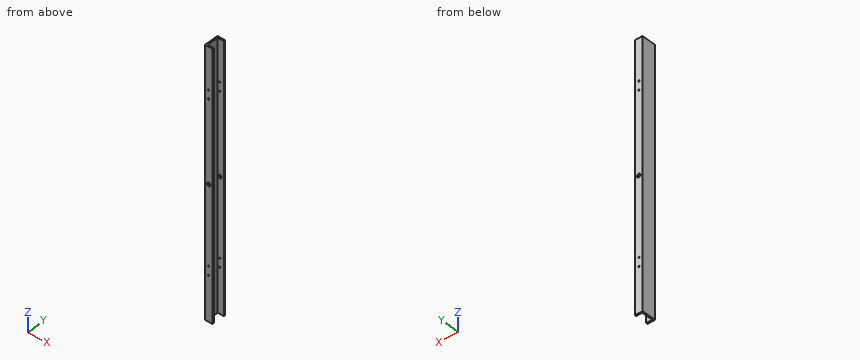
from build123d import *

# Parameters (mm, degrees)
BOSS_EXTRUDE1_DEPTH = 1360
SKETCH2_R           = 3.5
SKETCH2_R_2         = 9
CUT_EXTRUDE1_DEPTH  = 814.403343981


with BuildPart() as part:
    # Sketch1 → Boss-Extrude1 (new body)
    with BuildSketch(Plane.XY.offset(-680)):
        Polygon((-440, 550), (-440, 625), (-400, 625), (-400, 617), (-432, 617), (-432, 558), (-400, 558), (-400, 550), align=None)
    extrude(amount=BOSS_EXTRUDE1_DEPTH)

    # Sketch2 → Cut-Extrude1 (cut, through all)
    with BuildSketch(Plane(origin=(0, 625, 0), x_dir=(1, 0, 0), z_dir=(0, 1, 0))):
        with Locations(Location((-421, -467, 0), (0, 0, 270))):
            Circle(SKETCH2_R)
        with Locations(Location((-421, -422, 0), (0, 0, 270))):
            Circle(SKETCH2_R)
        with Locations(Location((-420, 0, 0), (0, 0, 270))):
            Circle(SKETCH2_R_2)
        with Locations(Location((-421, 450, 0), (0, 0, 270))):
            Circle(SKETCH2_R)
        with Locations(Location((-421, 405, 0), (0, 0, 270))):
            Circle(SKETCH2_R)
    extrude(amount=-CUT_EXTRUDE1_DEPTH, mode=Mode.SUBTRACT)


solid = part.part
The model under review builds one solid part; all positions refer to its coordinate system, in mm. Coordinates: 2 decimals unless noted, no trailing zeros. Loops run counter-clockwise (first coordinate to the right, second up) from the corner with the lowest first, then second, coordinate; pieces in that order, holes last. Notation, with made-up numbers: M -10.5,-29.75 L 32.5,-29.75 A17 ccw 32.5,1.25 Z; hole C -23,75 d4. An arc over 180 degrees is marked long. Put each result on its own line as item: value. Start each with the question number.
Q1. Add section B-B (y = 597.5). Write out the cut boundary in (x, z).
Q2. Clearance check with flat-ended pins moving along their axes: pin 1 (3 mm diameter, centred on y = 602.5, z = -86, fed in from +X); pin 2 (9 mm diameter, centred on x = -421, z = -450, fed in from +Y). State where each tip first meets the part, or that it passes through.
Q3. Add section A-A (z = 230). Write out the cut boundary in (x, y).
Q4. Wall thickness on line 1 (Z direction, x = -421, y = 621.25); line 2 (X direction, y = 619.75, z = -450); line 3 (Y direction, x = -404.5, z = 479.5): over which ranges is each line inside the solid? List them lowest first.
Answers:
1. outline: M -440,-680 L -432,-680 L -432,680 L -440,680 Z
2. pin 1: stops at x = -432
2. pin 2: stops at y = 625
3. outline: M -440,550 L -400,550 L -400,558 L -432,558 L -432,617 L -400,617 L -400,625 L -440,625 Z
4. line 1: z = -680 to -453.5, -446.5 to -408.5, -401.5 to -8.94, 8.94 to 418.5, 425.5 to 463.5, 470.5 to 680
4. line 2: x = -440 to -424.5, -417.5 to -400
4. line 3: y = 550 to 558, 617 to 625
